Could you check a few things on this model? Use its own coordinates, in mm. A direction names the side the tool comes from. Round coordinates to 2 decimals unless told otherwise and drop trailing zeros. Loops run counter-clockwise (first coordinate to the right, second up) from the corner with the lowest first, then second, coordinate; pieces in that order, holes last. Notation, with made-up numbers: M 61,13.5 L 78,13.5 A21 ccw 78,23.5 Z; hole C 54,-37.75 d7. An arc over 180 degrees is marked long. Answer in a Markdown table with one row per item.
```python
from build123d import *

# Parameters (mm, degrees)
CYLINDER_R     = 2.3
CYLINDER_DEPTH = 50
ARRAY_Z_COUNT  = 4
ARRAY_Z_PITCH  = 15
BOX_W          = 40
BOX_H          = 15
BOX_DEPTH      = 3
BOX002_W       = 4
BOX002_H       = 15
BOX002_DEPTH   = 50
FILLET_R       = 5
BOX001_W       = 3
BOX001_H       = 15
BOX001_DEPTH   = 15
FILLET001_R    = 4


with BuildPart() as bolt_hole_array:
    # Cylinder → Cylinder (new body)
    with BuildSketch(Plane(origin=(25, -1.3, -7), x_dir=(0, 0, 1), z_dir=(-1, 0, 0))):
        Circle(CYLINDER_R)
    extrude(amount=CYLINDER_DEPTH)

    # Array Z: bolt hole array ×4


with BuildPart() as bolt_hole_array_1:
    add(bolt_hole_array.part)
    with Locations(*[(0, 0, i * ARRAY_Z_PITCH) for i in range(1, ARRAY_Z_COUNT)]):
        add(bolt_hole_array.part)


with BuildPart() as top_panel:
    # Box → Box (new body)
    with BuildSketch(Plane(origin=(-20, -7.5, 0), x_dir=(1, 0, 0), z_dir=(0, 0, 1))):
        with Locations((20, 7.5)):
            Rectangle(BOX_W, BOX_H)
    extrude(amount=BOX_DEPTH)


with BuildPart() as vertical_cube_fillet:
    # Box002 → Box002 (new body)
    with BuildSketch(Plane(origin=(5, -7.5, 0), x_dir=(1, 0, 0), z_dir=(0, 0, 1))):
        with Locations((2, 7.5)):
            Rectangle(BOX002_W, BOX002_H)
    extrude(amount=BOX002_DEPTH)

    # Fillet
    fillet_edges = [vertical_cube_fillet.edges().sort_by_distance(p)[0] for p in [
        (7, -7.5, 50),
        (7, 7.5, 50),
    ]]
    fillet(fillet_edges, radius=FILLET_R)


with BuildPart() as part_mirroring001:
    # Part__Mirroring001: instance of vertical cube fillet
    add(vertical_cube_fillet.part.mirror(Plane(origin=(0, 0, 0), x_dir=(0, -1, 0), z_dir=(1, 0, 0))))


with BuildPart() as side_cube_fillet:
    # Box001 → Box001 (new body)
    with BuildSketch(Plane(origin=(20, -7.5, -12), x_dir=(1, 0, 0), z_dir=(0, 0, 1))):
        with Locations((1.5, 7.5)):
            Rectangle(BOX001_W, BOX001_H)
    extrude(amount=BOX001_DEPTH)

    # Fillet001
    fillet001_edges = [side_cube_fillet.edges().sort_by_distance(p)[0] for p in [
        (21.5, -7.5, -12),
        (21.5, 7.5, -12),
    ]]
    fillet(fillet001_edges, radius=FILLET001_R)


with BuildPart() as wire_holder_cut:
    # Part__Mirroring: instance of side cube fillet
    add(side_cube_fillet.part.mirror(Plane(origin=(0, 0, 0), x_dir=(0, -1, 0), z_dir=(1, 0, 0))))

    # Fusion: union top panel, Part__Mirroring001, vertical cube fillet, side cube fillet
    add(top_panel.part)
    add(part_mirroring001.part)
    add(vertical_cube_fillet.part)
    add(side_cube_fillet.part)

    # Cut: cut bolt hole array
    add(bolt_hole_array_1.part, mode=Mode.SUBTRACT)


solid = wire_holder_cut.part
```
1) I need wall thicknesses on line 1 (Z direction, x = 6.1, y = -1.3); line 2 (Z direction, x = -21.35, y = -1.3); line 3 (X direction, y = -3.5, z = 45.5). Which ranges of each line are inside material? Lowest first, please.
Computed:
| item | result |
|---|---|
| line 1 | z = 0 to 5.7, 10.3 to 20.7, 25.3 to 35.7, 40.3 to 50 |
| line 2 | z = -12 to -9.3, -4.7 to 3 |
| line 3 | x = -9 to -5, 5 to 9 |
2) I want a section at C-C, the plane x = -8. Please give me the cut outline in (y, z).
Computed:
| item | result |
|---|---|
| outline | M -7.5,0 L 7.5,0 L 7.5,45 A5 ccw 2.5,50 L -2.5,50 A5 ccw -7.5,45 Z; hole C -1.3,8 d4.6; hole C -1.3,23 d4.6; hole C -1.3,38 d4.6 |
3) If we mould it in two halves opening along Y, with no side actions, what happens to faces 5 (the face through (-5.2, -7.5, 14.5)), 6 (the face through (-7, 0, 50)), 7 (the face through (-6.972, -0.609, 25.194))? For each: released by +Y, released by -Y, zero draft, split by the parting line, or undercut.
Computed:
| item | result |
|---|---|
| face 5 | released by -Y |
| face 6 | zero draft |
| face 7 | undercut |
4) I want a section at B-B, the plane z = -7. Please give me the cut outline in (x, y).
Computed:
| item | result |
|---|---|
| outline | M -23,-7.5 L -20,-7.5 L -20,-3.6 L -23,-3.6 Z; M -23,1 L -20,1 L -20,7.5 L -23,7.5 Z; M 20,-7.5 L 23,-7.5 L 23,-3.6 L 20,-3.6 Z; M 20,1 L 23,1 L 23,7.5 L 20,7.5 Z |
5) I want a section at D-D, the plane y = -1.3. State how many separate pieces and enclosed holes the cut face has, plus the area to 3 significant figures.
Computed:
| item | result |
|---|---|
| separate pieces | 9 |
| enclosed holes | 0 |
| area | 448 mm² |
6) Will these pins go through, and if not, where does the flat tip stop? P1, Ø7.5, axis at y = 2, z = 18, coming from the +X side; P2, Ø5, axis at y = -0.5, z = 27, coming from the -X side; P3, Ø3, axis at x = -1, y = 1.5, coming from the +Z side.
Computed:
| item | result |
|---|---|
| P1 | stops at x = 9 |
| P2 | stops at x = -9 |
| P3 | stops at z = 3 |
7) Which directions (+Z, -Z, +X, -X, +Y, -Y) give clear straight access to the entire face, cutting with the end or side of a thin tool? Please do faces 1 (the face through (0, 0, 0)), 2 (the face through (-16, 0, 3)), 3 (the face through (16, 0, 3)), 4 (the face through (23, -0.1, -4.6)).
Computed:
| item | result |
|---|---|
| face 1 | -Z, +Y, -Y |
| face 2 | +Z, -X, +Y, -Y |
| face 3 | +Z, +X, +Y, -Y |
| face 4 | +Z, -Z, +X, +Y, -Y |
8) I want a section at A-A, the plane z = 41. Please give me the cut outline in (x, y), plus the area to 3 significant figures.
Computed:
| item | result |
|---|---|
| outline | M -9,-7.5 L -5,-7.5 L -5,7.5 L -9,7.5 Z; M 5,-7.5 L 9,-7.5 L 9,7.5 L 5,7.5 Z |
| area | 120 mm² |
